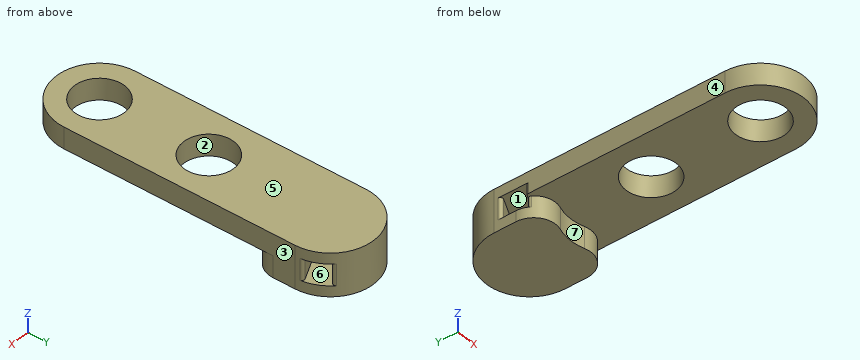
```python
from build123d import *

# Parameters (mm, degrees)
SKETCH3_R               = 1.8414999999999992
SKETCH3_R_2             = 1.8415000000000015
BOSS_EXTRUDE1_DEPTH     = 1.5875
BOSS_EXTRUDE2_START     = -1.5875
SKETCH3_3_R             = 3.1750000000000016
BOSS_EXTRUDE2_DEPTH     = 1.5875
CUT_EXTRUDE1_DEPTH      = 1.5875
CUT_EXTRUDE3_DEPTH      = 14.458066723062892
CUT_EXTRUDE3_DEPTH_BACK = 14.458066723062892
SKETCH9_W               = 1.5874999999999995
SKETCH9_H               = 1.5875000000000021
FILLET1_R               = 1.5875
FILLET3_R               = 0.19845020000000002


with BuildPart() as part:
    # Sketch3 → Boss-Extrude1 (new body)
    with BuildSketch(Plane.XY):
        with BuildLine():
            ThreePointArc((11.11246472217867, 0.03175000000000093), (14.287464722178669, -3.1432499999999988), (17.46246472217867, 0.03174999999999976))
            Line((17.46246472217867, 0.03175000000000054), (17.46246472217867, 16.668750000000003))
            ThreePointArc((17.46246472217867, 16.668750000000003), (14.287464722178667, 19.843750000000004), (11.112464722178665, 16.668750000000003))
            Line((11.112464722178666, 16.668750000000003), (11.11246472217867, 0.03174999999999883))
        make_face()
        with Locations((14.287464722178665, 7.905750000000001)):
            Circle(SKETCH3_R, mode=Mode.SUBTRACT)
        with Locations((14.287464722178669, 0.03175000000000054)):
            Circle(SKETCH3_R_2, mode=Mode.SUBTRACT)
    extrude(amount=BOSS_EXTRUDE1_DEPTH)

    # Sketch3<3> → Boss-Extrude2 (add)
    with BuildSketch(Plane.XY.offset(BOSS_EXTRUDE2_START)):
        with BuildLine():
            Line((14.287464727919362, 13.493750000000004), (17.46246472217867, 13.493750000000004))
            Line((17.46246472217867, 13.493750000000004), (17.46246472217867, 16.668750000000003))
            ThreePointArc((17.46246472217867, 16.668750000000003), (16.5325287544756, 14.423685971762355), (14.287464727919362, 13.493750000000002))
        make_face()
        with BuildLine():
            Line((11.11246472217867, 13.493750000000004), (14.287464727919362, 13.493750000000004))
            ThreePointArc((14.287464727919362, 13.493750000000002), (12.042400693941019, 14.423685967703072), (11.112464722178665, 16.668750000000003))
            Line((11.112464722178666, 16.668750000000003), (11.11246472217867, 13.493750000000004))
        make_face()
        with Locations((14.287464722178667, 16.668750000000003)):
            Circle(SKETCH3_3_R)
        with BuildLine():
            ThreePointArc((11.112464722178665, 10.318750009292732), (12.042400697226496, 12.56381403558241), (14.287464727919362, 13.493750000000002))
            Line((14.287464727919362, 13.493750000000004), (11.11246472217867, 13.493750000000004))
            Line((11.11246472217867, 13.493750000000004), (11.11246472217867, 10.318750009292732))
        make_face()
        with BuildLine():
            ThreePointArc((14.287464727919362, 13.493750000000002), (16.532528754475596, 12.563814028237648), (17.462464722178666, 10.318750000000003))
            Line((17.46246472217867, 10.318750000000003), (17.46246472217867, 13.493750000000004))
            Line((17.46246472217867, 13.493750000000004), (14.287464727919362, 13.493750000000004))
        make_face()
    extrude(amount=BOSS_EXTRUDE2_DEPTH)

    # Sketch4 → Cut-Extrude1 (cut)
    with BuildSketch(Plane(origin=(0, 0, -1.5875), x_dir=(-1, 0, 0), z_dir=(0, 0, -1))):
        with BuildLine():
            ThreePointArc((-11.366464722178668, 12.114801224213839), (-14.28746472217867, 13.747750000000003), (-17.208464722178668, 12.11480122421383))
            ThreePointArc((-17.208464722178668, 12.11480122421383), (-17.345736990888724, 11.869560023967814), (-17.4624647221787, 11.613900956452488))
            Line((-17.46246472217867, 11.613900956452483), (-17.46246472217867, 10.318750000000003))
            ThreePointArc((-17.46246472217867, 10.318750000000005), (-14.287464722178669, 13.493750000000002), (-11.112464722178668, 10.318750000000003))
            Line((-11.112464722178666, 10.318750000000003), (-11.112464722178666, 11.613900956452593))
            ThreePointArc((-11.112464722178673, 11.613900956452591), (-11.229192453468636, 11.86956002396787), (-11.366464722178668, 12.114801224213839))
        make_face()
        with BuildLine():
            Line((-17.46246472217867, 10.318750000000003), (-17.46246472217867, 11.613900956452483))
            ThreePointArc((-17.4624647221787, 11.613900956452488), (-14.947376079862362, 6.9538491099290844), (-10.858464722178665, 10.318750000000003))
            ThreePointArc((-10.858464722178665, 10.318750000000003), (-10.922563832107757, 10.978661357683757), (-11.112464722178673, 11.613900956452591))
            Line((-11.112464722178666, 11.613900956452593), (-11.112464722178666, 10.318750000000003))
            ThreePointArc((-11.112464722178668, 10.318750000000003), (-14.287464722178669, 13.493750000000002), (-17.46246472217867, 10.318750000000005))
        make_face()
    extrude(amount=-CUT_EXTRUDE1_DEPTH, mode=Mode.SUBTRACT)

    # Sketch9 → Cut-Extrude3 (cut, two sides: drawn at the far end of the back side and taken through both)
    with BuildSketch(Plane(origin=(14.949330355898779, 7.042270953374606, 0), x_dir=(0, 0, 1), z_dir=(-0.9046486230783365, -0.42615826726988393, 0)).offset(-CUT_EXTRUDE3_DEPTH_BACK)):
        with Locations((-1.1e-16, 9.003381908558007)):
            Rectangle(SKETCH9_W, SKETCH9_H)
    extrude(amount=CUT_EXTRUDE3_DEPTH + CUT_EXTRUDE3_DEPTH_BACK, mode=Mode.SUBTRACT)

    # Fillet1
    # the kernel refuses this fillet: 1.5875 mm, written as the material it takes off along each edge
    with BuildSketch(Plane(origin=(11.112464722178668, 11.613900956452579, 0), x_dir=(-5.1e-16, 1, 0), z_dir=(0, 0, -1))) as fillet1_piece_1:
        with BuildLine():
            CenterArc((3.463537518327043, 1.5875000000000004), FILLET1_R, 161.5512847696779, 108.44871523032214)
            ThreePointArc((1.9576234440297167, 2.0898734177215426), (1.2074075320922062, 0.8308067461464439), (0, 0))
            Line((0, 0), (3.463537518327044, 0))
        make_face()
    extrude(amount=10.24634379581761, mode=Mode.SUBTRACT)
    with BuildSketch(Plane(origin=(17.46246472217867, 11.613900956453127, 0), x_dir=(0, 1, 0), z_dir=(0, 0, -1))) as fillet1_piece_2:
        with BuildLine():
            CenterArc((3.4635375183265698, -1.5875000000000004), FILLET1_R, 90, 108.44871523031935)
            ThreePointArc((1.9576234440292186, -2.0898734177214706), (1.2074075320919153, -0.8308067461464965), (0, 0))
            Line((0, 0), (3.4635375183265698, 0))
        make_face()
    extrude(amount=10.246343795816424, mode=Mode.SUBTRACT)

    # Fillet3
    fillet3_edges = [part.edges().sort_by_distance(p)[0] for p in [
        (16.72182330744723, 18.70701477139974, -1.1e-16),
        (17.404301856828425, 17.273689068062478, -1.1e-16),
        (11.112464722178666, 14.309755511050398, 0.3968749999999998),
        (11.112464722178666, 16.064580488949616, -1.1e-16),
        (11.271579474224783, 14.38471065418466, -0.3968749999999999),
    ]]
    fillet(fillet3_edges, radius=FILLET3_R)


solid = part.part
```
Part model, mm, in its own coordinate system. Face numbers are marked on the shaded views. A direction names the side the tool comes from. Round coordinates to 2 decimals unless told otherwise and drop trailing zeros. Loops run counter-clockwise (first coordinate to the right, second up) from the corner with the lowest first, then second, coordinate; pieces in that order, holes last.
Item 1: Cut at D-D, the plane x = 12.25. Give the cut face in (y, z), then the cut area to 3 significant figures.
Item 2: Drill centre lines: line 1 (Y direction, x = 15.5, z = 0.6); line 2 (Y direction, x = 15.25, z = 0.7); line 3 (Z direction, x = 13, y = 15.25). Where is each one in solid material? Low to high.
Item 3: 3-axis set-ups, long thin cutter, end or side, ignore diameter. For the marked faces 5, 6 and 7: which of +Z, -Z, +X, -X, +Y, -Y reach the whole face in a straight line?
Item 4: Cut at A-A, the plane z = 0.6. State how many separate pieces and enclosed holes the cut face has, then the cut area to 3 significant figures.
Item 5: Mould opens along X. For the marked faces 1, 2, 3 and 4 say: +X half, -X half, draft (parallel to the pull), parting line (faces both ways), or undercut.
Item 6: Cut at B-B, the plane x = 14.75. Give the cut face in (y, z), then the cut area to 3 significant figures.
Item 7: Cut at C-C, the plane y = 9.5. Give the cut face in (x, z).
Item 8: Drop a flat-ended pin along its axis: P1, Ø1, axis at x = 15, y = 7.5, coming from the +Z side. Give the stop position or say it passes through.
A:
1. outline: (-2.4, 0) - (13.56, 0) - (13.56, -1.59) - (19.1, -1.59) - (19.1, 1.59) - (-2.4, 1.59) - close; hole (14.85, -0.79) - (16.6, -0.79) - (16.6, 0.79) - (14.85, 0.79) - close
1. area: 40.2 mm2
2. line 1: y = -2.9 to -1.35, 1.42 to 6.52, 9.29 to 16.38, 18.13 to 19.6
2. line 2: y = -2.99 to -1.54, 1.6 to 6.34, 9.48 to 16.26, 18.01 to 19.69
2. line 3: z = -1.59 to -0.79, 0.79 to 1.59
3. face 5: +Z, +X, -X, +Y, -Y
3. face 6: none
3. face 7: -Z, -Y
4. separate pieces: 2
4. enclosed holes: 2
4. area: 105 mm2
5. face 1: undercut
5. face 2: undercut
5. face 3: +X half
5. face 4: -X half
6. outline: (-3.11, 0) - (-1.75, 0) - (-1.75, 1.59) - (-3.11, 1.59) - close; (1.81, 0) - (6.12, 0) - (6.12, 1.59) - (1.81, 1.59) - close; (9.69, 0) - (13.72, 0) - (13.72, -1.59) - (19.81, -1.59) - (19.81, 1.59) - (9.69, 1.59) - close; hole (16.02, -0.79) - (17.78, -0.79) - (17.78, 0.79) - (16.02, 0.79) - close
6. area: 32.0 mm2
7. outline: (11.11, 0) - (13.37, 0) - (13.37, 1.59) - (11.11, 1.59) - close; (15.21, 0) - (17.46, 0) - (17.46, 1.59) - (15.21, 1.59) - close
8. P1: passes through
